from build123d import *

# Parameters (mm, degrees)
F0_W      = 80.9689760208
F0_H      = 136.9662135839
F1_DEPTH  = 7.366
F2_R      = 5.08
F3_W      = 70.8160358799
F3_H      = 119.3651366365
F4_DEPTH  = 0.508
F5_R      = 4.2062537649
F6_DEPTH  = 0.762
F7_W      = 9.7111202776
F7_H      = 2.8320385609
F8_DEPTH  = 2.54
F9_R      = 2.3153657449
F10_DEPTH = 1.6256
F11_R     = 2.4503430009
F12_DEPTH = 1.778
F14_R     = 3.8927406251
F15_DEPTH = 1.524
F16_R     = 1.7892494252
F17_DEPTH = 4.064
F18_R     = 0.6717284453
F19_DEPTH = 5.08
F21_DEPTH = 3.302
F22_R     = 2.1300534038
F23_DEPTH = 6.858


with BuildPart() as f1:
    # F0 (on Top) → F1 (new body)
    with BuildSketch(Plane.XY):
        with Locations((0.3460086882, -4.4899731874)):
            Rectangle(F0_W, F0_H)
    extrude(amount=F1_DEPTH)

    # F2
    f2_edges = [f1.edges().sort_by_distance(p)[0] for p in [
        (-40.138479, 63.993134, 3.683),
        (40.830497, 63.993134, 3.683),
        (40.830497, -72.97308, 3.683),
        (-40.138479, -72.97308, 3.683),
    ]]
    fillet(f2_edges, radius=F2_R)

    # F3 (on face) → F4 (cut)
    with BuildSketch(Plane.XY.offset(7.366)):
        with Locations((0.3495386177, -0.7694347137)):
            Rectangle(F3_W, F3_H)
    extrude(amount=-F4_DEPTH, mode=Mode.SUBTRACT)

    # F5 (on face) → F6 (cut)
    with BuildSketch(Plane.XY.offset(7.366)):
        with Locations((0, -65.5538588762)):
            Circle(F5_R)
    extrude(amount=-F6_DEPTH, mode=Mode.SUBTRACT)

    # F7 (on face) → F8 (cut)
    with BuildSketch(Plane(origin=(-40.1384793222, 0, 0), x_dir=(0, -1, 0), z_dir=(-1, 0, 0))):
        with Locations((-42.3318911344, 3.4466114594)):
            Rectangle(F7_W, F7_H)
    extrude(amount=-F8_DEPTH, mode=Mode.SUBTRACT)

    # F9 (on face) → F10 (join)
    with BuildSketch(Plane(origin=(-40.1384793222, 0, 0), x_dir=(0, -1, 0), z_dir=(-1, 0, 0))):
        with Locations((-31.1954244971, 3.375432454)):
            Circle(F9_R)
    extrude(amount=F10_DEPTH)

    # F11 (on face) → F12 (join)
    with BuildSketch(Plane(origin=(-40.1384793222, 0, 0), x_dir=(0, -1, 0), z_dir=(-1, 0, 0))):
        with Locations((-22.7978900075, 3.2298590522)):
            Circle(F11_R)
    extrude(amount=F12_DEPTH)

    # F14 (on face) → F15 (cut)
    with BuildSketch(Plane(origin=(0, 0, 0), x_dir=(1, 0, 0), z_dir=(0, 0, -1))):
        with Locations((31.0994051397, -53.9800077677)):
            Circle(F14_R)
    extrude(amount=-F15_DEPTH, mode=Mode.SUBTRACT)

    # F16 (on face) → F17 (cut)
    with BuildSketch(Plane(origin=(0, 0, 0), x_dir=(1, 0, 0), z_dir=(0, 0, -1))):
        with Locations((31.2404166907, -54.5385442674)):
            Circle(F16_R)
    extrude(amount=-F17_DEPTH, mode=Mode.SUBTRACT)

    # F18 (on face) → F19 (cut)
    with BuildSketch(Plane(origin=(0, 0, 0), x_dir=(1, 0, 0), z_dir=(0, 0, -1))):
        with Locations((24.6018432081, -55.6784830987)):
            Circle(F18_R)
    extrude(amount=-F19_DEPTH, mode=Mode.SUBTRACT)

    # F20 (on face) → F21 (cut)
    with BuildSketch(Plane(origin=(0, 0, 0), x_dir=(1, 0, 0), z_dir=(0, 0, -1))):
        with BuildLine():
            add(Edge.make_bspline(
                [(21.838599816, -57.1239739656), (22.3255501081, -55.7146974508), (22.4935564689, -52.3704464682), (19.2282519734, -51.1257918433), (17.6040761183, -53.0174394253), (17.5519956723, -57.9087722175), (20.2838683925, -59.75590869), (21.4647452863, -58.2059415034), (21.838599816, -57.1239739656)],
                knots=[0, 0, 0, 0, 0.2013997834, 0.354787719, 0.491355532, 0.6980279839, 0.8453759603, 1, 1, 1, 1], degree=3))
        make_face()
    extrude(amount=-F21_DEPTH, mode=Mode.SUBTRACT)

    # F22 (on face) → F23 (cut)
    with BuildSketch(Plane.XZ.offset(72.9730799794)):
        with Locations((-16.7610161006, 3.8362841588)):
            Circle(F22_R)
    extrude(amount=-F23_DEPTH, mode=Mode.SUBTRACT)


solid = f1.part
Can you work these out from the model? Positions are in its coordinate system, mm. A direction names the side the tool comes from. Round coordinates to 2 decimals unless told otherwise and drop trailing zeros. Write each loop counter-clockwise with the first axis right and the second up, starting at its lowest first coordinate (ties: lowest second). Pieces come first, ordered by that corner, then holes. Notation, with made-up numbers: (29, -21) -> (35, -21) arc R18 ccw to (35, -8) -> close; hole circle Ø9 at (17.25, -29). An arc over 180 degrees is marked (long way). Use one line per item in the form item = value. Start each with the question number.
Q1. Imagine slicing it at A-A (y = -55.5). Please give me the cut outline in (x, z).
Q2. We'd pull the mould along X, two halves only. Please class faces 6 (the face through (-37.598, 42, 3)), 7 (the face through (30, 53, 1.524)), 8 (the face through (-17, -66.115, 4)), 9 (the face through (-36, -14, 7.366)): +X half, -X half, draft (parallel to the pull), parting line (faces both ways), or undercut.
Q3. Imagine slicing it at D-D (y = 23). Please give me the cut outline in (x, z), then the cut area to 3 significant figures.
Q4. Which directions (+Z, -Z, +X, -X, +Y, -Y) give clear straight access to the entire face, cutting with the end or side of a thin tool? Please do faces 1 (the face through (-39, 42, 2.031)), 2 (the face through (39.38, 62.47, 3.73)), 3 (the face through (0, 63.993, 4)), 4 (the face through (30.59, 50.12, 0.75)), 5 (the face through (2.261, -62.007, 6.99)).
Q5. Imagine slicing it at C-C (x = -27.5). Please give me the cut outline in (y, z).
Q6. I'm going to push flat-ended pins straight in: P1, Ø21, axis at x = 12.5, y = 20, coming from the +Z side; P2, Ø1.4, axis at y = 42.5, z = 3.5, coming from the -X side; P3, Ø2, axis at x = -39, z = 4, coming from the -Y side. Where does each tip first touch, or does it pass through?
Q7. If I drill on probe 1 along X at (y, z) = (54.5, 4); probe 2 along Z at (x, y) = (-4.5, 53.5); probe 3 along X at (y, z) = (-4, 2.5), over which ranges is the centre line in solid material (lowest first)? Write a range as [from, to].
Q8. Imagine slicing it at B-B (x = 0). Please give me the cut outline in (y, z), then the cut area to 3 significant figures.
Worked out:
q1.outline = (-40.14, 0) -> (40.83, 0) -> (40.83, 7.37) -> (35.76, 7.37) -> (35.76, 6.86) -> (-35.06, 6.86) -> (-35.06, 7.37) -> (-40.14, 7.37) -> close
q2.face_6 = -X half
q2.face_7 = undercut
q2.face_8 = undercut
q2.face_9 = draft
q3.outline = (-41.92, 0.79) -> (-40.14, 0.79) -> (-40.14, 0) -> (40.83, 0) -> (40.83, 7.37) -> (35.76, 7.37) -> (35.76, 6.86) -> (-35.06, 6.86) -> (-35.06, 7.37) -> (-40.14, 7.37) -> (-40.14, 5.67) -> (-41.92, 5.67) -> close
q3.area = 569 mm^2
q4.face_1 = -X
q4.face_2 = +Z, -Z, +X, +Y
q4.face_3 = +Z, -Z, +X, -X, +Y
q4.face_4 = -Z
q4.face_5 = +Z
q5.outline = (-72.97, 0) -> (63.99, 0) -> (63.99, 7.37) -> (58.91, 7.37) -> (58.91, 6.86) -> (-60.45, 6.86) -> (-60.45, 7.37) -> (-72.97, 7.37) -> close
q6.P1 = 6.86
q6.P2 = -37.6
q6.P3 = -72.03
q7.probe_1 = [-40.14, 29.45], [33.03, 40.83]
q7.probe_2 = [0, 6.86]
q7.probe_3 = [-40.14, 40.83]
q8.outline = (-72.97, 0) -> (63.99, 0) -> (63.99, 7.37) -> (58.91, 7.37) -> (58.91, 6.86) -> (-60.45, 6.86) -> (-60.45, 7.37) -> (-61.35, 7.37) -> (-61.35, 6.6) -> (-69.76, 6.6) -> (-69.76, 7.37) -> (-72.97, 7.37) -> close
q8.area = 942 mm^2
